Work out the finished part from the listing and answer in its coordinate system (mm). Coordinates: 2 decimals unless noted, no trailing zeros. Order: outer loops, then holes, each group sorted by start corner. A loop starts at its lowest first (then second) coordinate and runs counter-clockwise, first axis right, second up.
1. The part is cut by section D-D, the plane x = 0. Give the vertices of the cut face in (y, z), then the cut area to 3 significant figures.
2. The part is cut by section A-A, the plane x = -15. Give the vertices of the cut face in (y, z).
3. Find the intervals of material crossed by probe 1 along Y at (x, z) = (15, 3.05); probe 2 along Y at (x, z) = (0, 0.55); probe 3 along Y at (x, z) = (-16, 1.9), in increasing order.
4. The part is cut by section C-C, the plane z = 3. Give the vertices of the cut face in (x, y), then the cut area to 3 significant figures.
```python
from build123d import *

# Parameters (mm, degrees)
SKETCH1_W           = 40
SKETCH1_H           = 40
BOSS_EXTRUDE1_DEPTH = 4
SKETCH2_R           = 2
CUT_EXTRUDE1_DEPTH  = 4
SKETCH3_R           = 2
CUT_EXTRUDE2_DEPTH  = 4


with BuildPart() as part:
    # Sketch1 → Boss-Extrude1 (new body)
    with BuildSketch(Plane.XY):
        Rectangle(SKETCH1_W, SKETCH1_H)
    extrude(amount=BOSS_EXTRUDE1_DEPTH)

    # Sketch2 → Cut-Extrude1 (cut)
    with BuildSketch(Plane.XY.offset(4)):
        with Locations((-15, 15)):
            Circle(SKETCH2_R)
        with Locations((15, 15)):
            Circle(SKETCH2_R)
        with Locations((15, -15)):
            Circle(SKETCH2_R)
        with Locations((-15, -15)):
            Circle(SKETCH2_R)
    extrude(amount=-CUT_EXTRUDE1_DEPTH, mode=Mode.SUBTRACT)

    # Sketch3 → Cut-Extrude2 (cut)
    with BuildSketch(Plane.XY.offset(4)):
        Circle(SKETCH3_R)
    extrude(amount=-CUT_EXTRUDE2_DEPTH, mode=Mode.SUBTRACT)


solid = part.part
```
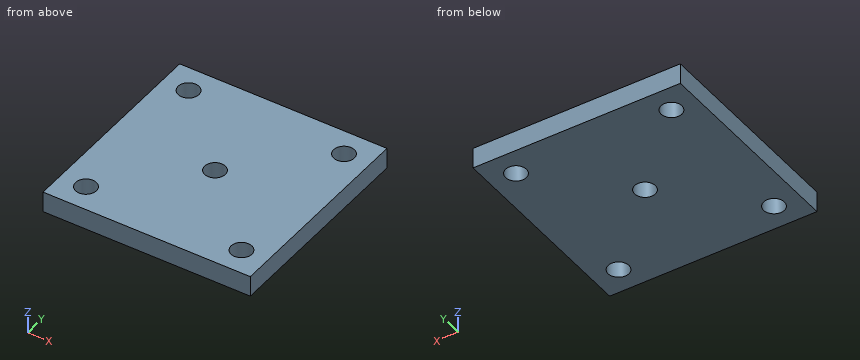
Geometry says:
1. outline: (-20, 0) - (-2, 0) - (-2, 4) - (-20, 4) - close; (2, 0) - (20, 0) - (20, 4) - (2, 4) - close
1. area: 144 mm2
2. outline: (-20, 0) - (-17, 0) - (-17, 4) - (-20, 4) - close; (-13, 0) - (13, 0) - (13, 4) - (-13, 4) - close; (17, 0) - (20, 0) - (20, 4) - (17, 4) - close
3. probe 1: y = -20 to -17, -13 to 13, 17 to 20
3. probe 2: y = -20 to -2, 2 to 20
3. probe 3: y = -20 to -16.73, -13.27 to 13.27, 16.73 to 20
4. outline: (-20, -20) - (20, -20) - (20, 20) - (-20, 20) - close; hole circle Ø4 at (-15, -15); hole circle Ø4 at (-15, 15); hole circle Ø4 at (0, 0); hole circle Ø4 at (15, -15); hole circle Ø4 at (15, 15)
4. area: 1,540 mm2
